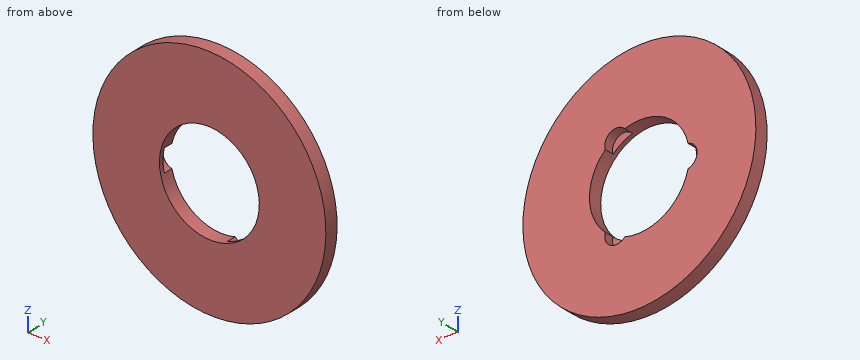
```python
from build123d import *

# Parameters (mm, degrees)
SKETCH1_R           = 70
BOSS_EXTRUDE1_DEPTH = 8
SKETCH2_R           = 30
CUT_EXTRUDE1_DEPTH  = 100.317672143
SKETCH3_R           = 6.888520525
CUT_EXTRUDE2_DEPTH  = 5.490022
CIRPATTERN1_START   = 2.509977764
CIRPATTERN1_DEPTH   = 5.490022236


# Read off the part's stored shape, not the designer's step: CirPattern1
with BuildPart() as part:
    # Sketch1 → Boss-Extrude1 (new body)
    with BuildSketch(Plane(origin=(0, 0, 0), x_dir=(1, 0, 0), z_dir=(0, 1, 0))):
        with Locations(Location((0, 0, 0), (0, 0, 270))):
            Circle(SKETCH1_R)
    extrude(amount=BOSS_EXTRUDE1_DEPTH)

    # Sketch2 → Cut-Extrude1 (cut, through all)
    with BuildSketch(Plane(origin=(0, 0, 0), x_dir=(1, 0, 0), z_dir=(0, 1, 0))):
        with Locations(Location((0, 0, 0), (0, 0, 270))):
            Circle(SKETCH2_R)
    extrude(amount=CUT_EXTRUDE1_DEPTH, mode=Mode.SUBTRACT)

    # Sketch3 → Cut-Extrude2 (cut)
    with BuildSketch(Plane(origin=(0, 8, 0), x_dir=(1, 0, 0), z_dir=(0, 1, 0))):
        with Locations((-27.809030926, 0)):
            Circle(SKETCH3_R)
    extrude(amount=-CUT_EXTRUDE2_DEPTH, mode=Mode.SUBTRACT)

    # CirPattern1 outline → CirPattern1 (cut)
    with BuildSketch(Plane(origin=(0, 0, 0), x_dir=(1, 0, 0), z_dir=(0, 1, 0)).offset(CIRPATTERN1_START)):
        with BuildLine():
            ThreePointArc((8.779812682, 28.68649315), (15, 25.980762114), (20.453325473, 21.946787398))
            ThreePointArc((20.453325473, 21.946787398), (17.348775725, 30.048961006), (8.779812682, 28.68649315))
        make_face()
        with BuildLine():
            ThreePointArc((20.453325473, -21.946787398), (15, -25.980762114), (8.779812682, -28.68649315))
            ThreePointArc((8.779812682, -28.68649315), (17.348775725, -30.048961006), (20.453325473, -21.946787398))
        make_face()
    extrude(amount=CIRPATTERN1_DEPTH, mode=Mode.SUBTRACT)


solid = part.part
```
Model file for the job. Use its own axes, mm. Coordinates: 2 decimals unless noted, no trailing zeros. Order: outer loops, then holes, each group sorted by start corner. A loop starts at its lowest first (then second) coordinate and runs counter-clockwise, first axis right, second up. Notation, with made-up numbers: (38.25, -24.75) -> (87.25, -24.75) arc R7 cw to (87.25, -17.75) -> close; hole circle Ø1 at (-13, -29). An arc over 180 degrees is marked (long way). Answer as a JSON object with one key per item and string values. Group by question number.
1) Cut at B-B, the plane x = 0. Write the cut outline in (y, z).
2) Cut at D-D, the plane z = -27. Write the cut outline in (x, y), then the cut area to 3 significant figures.
3) Cut at A-A, the plane z = 0. Write the cut outline in (x, y), then the cut area to 3 significant figures.
4) Drill centre lines: L1, parallel to X at y = 2, z = 0; L2, parallel to X at y = 6.5, z = 22; L3, parallel to Z at x = 25.5, y = 3.25. Where is each one in solid material? Low to high.
5) Flat gauge pins, fed straight in: pin 1 (2 mm diameter, centred on x = -4.5, y = 4, fed in from -Z); pin 2 (3 mm diameter, centred on x = -11.5, y = 4, fed in from -Z); pin 3 (7 mm diameter, centred on x = 15, z = 26.5, fed in from +Y). Where does each tip first touch, or does it go through?
6) Cut at C-C, the plane y = 5.5. Write the cut outline in (x, z).
Check values:
{
 "1": {"outline": "(0, -70) -> (8, -70) -> (8, -30) -> (0, -30) -> close; (0, 30) -> (8, 30) -> (8, 70) -> (0, 70) -> close"},
 "2": {"outline": "(-64.58, 0) -> (-13.08, 0) -> (-13.08, 8) -> (-64.58, 8) -> close; (13.08, 0) -> (64.58, 0) -> (64.58, 8) -> (20.15, 8) -> (20.15, 2.51) -> (13.08, 2.51) -> close", "area": "785 mm²"},
 "3": {"outline": "(-70, 0) -> (-30, 0) -> (-30, 2.51) -> (-34.7, 2.51) -> (-34.7, 8) -> (-70, 8) -> close; (30, 0) -> (70, 0) -> (70, 8) -> (30, 8) -> close", "area": "614 mm²"},
 "4": {"L1": "x = -70 to -30, 30 to 70", "L2": "x = -66.45 to -20.4, 20.47 to 66.45", "L3": "z = -65.19 to -15.8, 15.8 to 65.19"},
 "5": {"pin 1": "stops at z = -69.91", "pin 2": "stops at z = -69.28", "pin 3": "stops at y = 2.51"},
 "6": {"outline": "circle Ø140 at (0, 0); hole (-29.23, -6.74) arc R30 ccw to (8.78, -28.69) arc R6.89 ccw to (20.45, -21.95) arc R30 ccw to (20.45, 21.95) arc R6.89 ccw to (8.78, 28.69) arc R30 ccw to (-29.23, 6.74) arc R6.89 ccw to start"}
}
